from build123d import *

# Parameters (mm, degrees)
F1_DEPTH = 10
F2_SIZE2 = 24.99999
F2_SIZE  = 4.99999
F4_COUNT = 4
F5_W     = 60
F5_H     = 60
F5_W_2   = 50
F5_H_2   = 50
F6_DEPTH = 15
F8_DEPTH = 10
F9_DEPTH = 12


# Not quite as in the source:
# - a fillet or chamfer is up to 0.001 mm smaller than in the source, because OpenCascade refuses the exact size


with BuildPart() as f1:
    # F0 (on Top) → F1 (new body)
    with BuildSketch(Plane.XY):
        Polygon((-25, 0), (0, 0), (-25, 25), align=None)
        Polygon((-25, 25), (0, 0), (0, 25), align=None)
    extrude(amount=F1_DEPTH)

    # F2 (size 5 and 25 in the source; OpenCascade refuses exactly that, so slightly less here)
    f2_edges = [f1.edges().sort_by_distance(p)[0] for p in [
        (-12.5, 0, 10),
        (0, 12.5, 10),
    ]]
    chamfer(f2_edges, length=F2_SIZE, length2=F2_SIZE2)


with BuildPart() as f4_1:
    # F4: instance of F1
    add(f1.part.rotate(Axis((0, 0, -0.4458203912), (0, 0, -1)), 1 * 360 / F4_COUNT))


with BuildPart() as f4_2:
    # F4: instance of F1
    add(f1.part.rotate(Axis((0, 0, -0.4458203912), (0, 0, -1)), 2 * 360 / F4_COUNT))


with BuildPart() as f4_3:
    # F4: instance of F1
    add(f1.part.rotate(Axis((0, 0, -0.4458203912), (0, 0, -1)), 3 * 360 / F4_COUNT))


with BuildPart() as f1_1:
    add(f1.part)

    add(f4_1.part)  # F6 merges F4_1

    add(f4_2.part)  # F6 merges F4_2

    add(f4_3.part)  # F6 merges F4_3
    # F5 (on face) → F6 (join)
    with BuildSketch(Plane(origin=(0, 0, 0), x_dir=(1, 0, 0), z_dir=(0, 0, -1))):
        Rectangle(F5_W, F5_H)
        Rectangle(F5_W_2, F5_H_2, mode=Mode.SUBTRACT)
    extrude(amount=-F6_DEPTH)

    # F7 (on face) → F8 (cut)
    with BuildSketch(Plane.XY.offset(15)):
        Polygon((25, 25), (0, 25), (7.3223304703, 17.6776695297), (17.6776695297, 17.6776695297), (17.6776695297, 7.3223304703), (25, 0), align=None)
        Polygon((-7.3223304703, 17.6776695297), (0, 25), (-25, 25), (-25, 0), (-17.6776695297, 7.3223304703), (-17.6776695297, 17.6776695297), align=None)
        Polygon((-17.6776695297, -7.3223304703), (-25, 0), (-25, -25), (0, -25), (-7.3223304703, -17.6776695297), (-17.6776695297, -17.6776695297), align=None)
        Polygon((25, -25), (25, 0), (17.6776695297, -7.3223304703), (17.6776695297, -17.6776695297), (7.3223304703, -17.6776695297), (0, -25), align=None)
    extrude(amount=-F8_DEPTH, mode=Mode.SUBTRACT)

    # F9 (cut): a face of the model
    f9_faces = [f1_1.faces().sort_by_distance(p)[0] for p in [
        (0, 29.1514718626, 15),
    ]]
    extrude(f9_faces, amount=-F9_DEPTH, mode=Mode.SUBTRACT)


solid = f1_1.part
Read the model definition and answer for the solid it produces. Units are mm, in the model's axes. A direction names the side the tool comes from. Round coordinates to 2 decimals unless told otherwise and drop trailing zeros. Loops run counter-clockwise (first coordinate to the right, second up) from the corner with the lowest first, then second, coordinate; pieces in that order, holes last.
Q1. Each of these flat-tipped pins is pushed along its axis until it touches: pin 1 (12.5 mm diameter, centred on x = 13, y = -11.5, fed in from +Z); pin 2 (4 mm diameter, centred on x = 13, z = 4, fed in from +Y); pin 3 (1.1 mm diameter, centred on y = -13, z = 7.5, fed in from -X); pin 4 (3 mm diameter, centred on x = -12, z = 6, fed in from -Y). Where does it stop, or does it pass through?
Q2. Section C-C on x = 18.5 is taken. Write down the section's boundary in (y, z).
Q3. Section B-B on x = 5 is taken. Write down the section's boundary in (y, z), and give its area (3 significant figures).
Q4. Section D-D on y = -22 is taken. Write down the section's boundary in (x, z).
Q5. Section A-A on y = -13 is taken. Write down the section's boundary in (x, z), and give its area (3 significant figures).
Q6. Which of the six approach directions +Z, -Z, +X, -X, +Y, -Y give full straight-line access (tool end or side, diameter ignored) to faces 1 (the face through (-20.5, -4.5, 5.6)), 2 (the face through (-5, -13, 6)), 3 (the face through (12, 5, 6)), 4 (the face through (-15, 18, 5))?
Q7. Consider probe 1 along Z at (x, y) = (-19, -21); probe 2 along Z at (x, y) = (27, 14.5); probe 3 along X at (y, z) = (9, 4.5). Determine where each line is inside the solid, lowest interval first.
Q8. Determine the mould class of faces 5 (the face through (17.678, -14, 6)), 6 (the face through (5, -12, 6)), 7 (the face through (18, 18, 5)) for opening direction X: released by +X, released by -X, zero draft, split by the parting line, or undercut.
Output:
1. pin 1: stops at z = 8.32
1. pin 2: stops at y = 30
1. pin 3: stops at x = -17.68
1. pin 4: stops at y = -25
2. outline: (-30, 0) - (30, 0) - (30, 3) - (25, 3) - (25, 5) - (6.5, 5) - (6.5, 6.3) - (0, 5) - (-6.5, 6.3) - (-6.5, 5) - (-25, 5) - (-25, 3) - (-30, 3) - close
3. outline: (-30, 0) - (30, 0) - (30, 3) - (25, 3) - (25, 5) - (20, 5) - (20, 6) - (5, 6) - (0, 5) - (-5, 6) - (-20, 6) - (-20, 5) - (-25, 5) - (-25, 3) - (-30, 3) - close
3. area: 315 mm2
4. outline: (-30, 0) - (30, 0) - (30, 3) - (25, 3) - (25, 5) - (3, 5) - (3, 5.6) - (0, 5) - (-3, 5.6) - (-3, 5) - (-25, 5) - (-25, 3) - (-30, 3) - close
5. outline: (-30, 0) - (30, 0) - (30, 3) - (25, 3) - (25, 5) - (17.68, 5) - (17.68, 7.6) - (13, 7.6) - (0, 5) - (-13, 7.6) - (-17.68, 7.6) - (-17.68, 5) - (-25, 5) - (-25, 3) - (-30, 3) - close
5. area: 338 mm2
6. face 1: +Z, -X, -Y
6. face 2: +Z, +Y, -Y
6. face 3: +Z, +X, -X
6. face 4: +Z, -X, +Y
7. probe 1: z = 0 to 5
7. probe 2: z = 0 to 3
7. probe 3: x = -25 to 25
8. face 5: released by +X
8. face 6: undercut
8. face 7: zero draft
